The listing builds one solid part. Answer for the finished solid, in the listing's coordinates (mm). A direction names the side the tool comes from. Give positions to 0.01 mm unless a question says otherwise; leave off trailing zeros. Loops run counter-clockwise (first coordinate to the right, second up) from the corner with the lowest first, then second, coordinate; pieces in that order, holes last. Notation, with made-up numbers: M 85.5,-33 L 128.5,-33 A5 cw 128.5,-27 Z; hole C 26,71 d4. An arc over 180 degrees is marked long. Return JSON: item names as keys, results as strings.
Autodesk Inventor part; units mm, degrees
ref_plane "작업 평면1" through (0, 0, 0) normal (0, 0, 1) x (1, 0, 0)
ref_plane "YZ Plane" through (0, 0, 0) normal (1, 0, 0) x (0, 1, 0)
ref_plane "XZ Plane" through (0, 0, 0) normal (0, 1, 0) x (-1, 0, 0)
sketch "스케치1" plane through (0, 0, 0) normal (0, 0, 1) x (1, 0, 0)
  line L0 (0, 0) -> (24, 0)
  line L1 (24, 0) -> (24, -24)
  line L2 (24, -24) -> (0, -24)
  line L3 (0, -24) -> (0, 0)
  circle A0 centre (12, -12) radius 2.5
  dimension "d0" = 24
  dimension "d1" = 24
  dimension "d2" = 5
  dimension "d3" = 12
  dimension "d4" = 12
extrude "돌출1" add sketch "스케치1" along normal mid plane 35
fillet "모깎기1" radius 20 1 edges at (0, -24, 0)
chamfer "모따기1" distance 2 angle 45 4 edges at (12, 0, 17.5) (12, 0, -17.5) (24, -12, 17.5) (24, -12, -17.5)
ref_plane "작업 평면1" through (0, 0, 0) normal (0, 0, 1) x (1, 0, 0)
sketch "스케치2" plane through (0, 0, 0) normal (0, 0, 1) x (1, 0, 0)
  line L0 (24, -24) -> (24, 0)
  line L1 (24, 0) -> (20, 0)
  line L2 (20, 0) -> (20, -4)
  line L3 (20, -4) -> (24, -4)
  line L4 (24, -4) -> (24, 0)
  line L5 (0, 0) -> (0, -2)
  line L6 (0, 0) -> (4, 0)
  line L7 (4, 0) -> (4, -4)
  line L8 (4, -4) -> (0, -4)
  line L9 (0, -4) -> (0, 0)
  line L10 (22, -24) -> (24, -24)
  line L11 (24, -24) -> (20, -24)
  line L12 (20, -24) -> (20, -20)
  line L13 (20, -20) -> (24, -20)
  line L14 (24, -20) -> (24, -24)
  line L15 (22, -2) -> (24, 0)
  line L16 (24, 0) -> (0, 0)
  line L17 (0, 0) -> (0, -24)
  line L18 (0, -24) -> (24, -24)
  line L19 (24, -24) -> (24, 0)
  dimension "d11" = 4
  dimension "d12" = 4
  dimension "d13" = 4
  dimension "d14" = 4
  dimension "d15" = 4
extrude "돌출2" cut sketch "스케치2" along normal mid plane 27 contours L13 L12 L18 L17 L8 L7 L16 L2 L3 L0
properties part number "16-1"
(1) The part is cut by section C-C (y = -19). Determine the outline of the cut face in (x, z).
Values follow:
{"outline": "M 6.77,-17.5 L 22,-17.5 L 24,-15.5 L 24,-13.5 L 6.77,-13.5 Z; M 6.77,13.5 L 24,13.5 L 24,15.5 L 22,17.5 L 6.77,17.5 Z"}
(2) Given pin 1 (6 mm diameter, centred on x = 6, z = -8.5, fed in from -Y); pin 2 (4 mm diameter, centred on x = 12, y = -12, fed in from +Z); pin 3 (3 mm diameter, centred on y = -21.5, z = 0, fed in from -X), each flat-ended and moving along its own axis, determine where each tip first touches the part or whether it passes through.
Values follow:
{"pin 1": "y = -4", "pin 2": "through", "pin 3": "x = 20"}
(3) Determine the mould class of faces 4 (the flat face through (14, -9, -13.5)), 5 (the cylindrical face through (5.703, -17.986, 15.528)), 6 (the flat face through (23, -11.8, 16.5)) for opening direction Z: released by +Z, released by -Z, zero draft, split by the parting line, or undercut.
Values follow:
{"face 4": "undercut", "face 5": "zero draft", "face 6": "released by +Z"}
(4) Straight lines are drawn through the part: line 1 along Z through (x, y) = (7.75, -19.5); line 2 along Y through (x, z) = (2.25, 12.5); line 3 along Y through (x, z) = (12, -16.4). For each, find the intervals that lie inside material, in ascending order.
Values follow:
{"line 1": "-17.5 to -13.5, 13.5 to 17.5", "line 2": "-4 to 0", "line 3": "-22.33 to -14.5, -9.5 to -0.9"}
(5) The part is cut by section D-D (x = 4.5). Determine the outline of the cut face in (y, z).
Values follow:
{"outline": "M -16.64,-17.5 L -2,-17.5 L 0,-15.5 L 0,-13.5 L -16.64,-13.5 Z; M -16.64,13.5 L 0,13.5 L 0,15.5 L -2,17.5 L -16.64,17.5 Z"}
(6) The part is cut by section A-A (z = -6). Determine the outline of the cut face in (x, y), and give its area (3 significant figures).
Values follow:
{"outline": "M 0,-4 L 4,-4 L 4,0 L 0,0 Z; M 20,-24 L 24,-24 L 24,-20 L 20,-20 Z; M 20,-4 L 24,-4 L 24,0 L 20,0 Z", "area": "48.0 mm²"}
(7) A tool of negligible diameter and unlimited length cuts with its end or side. For faces 1 (the flat face through (4, -2, 0)), 2 (the flat face through (2, -4, 0)), 3 (the flat face through (22, -20, 0)), from which of +Z, -Z, +X, -X, +Y, -Y can it reach the whole face along a straight path? Write none if from no direction.
Values follow:
{"face 1": "+Y, -Y", "face 2": "+X, -X, -Y", "face 3": "+X, -X"}
(8) The part is cut by section B-B (x = 12). Determine the outline of the cut face in (y, z).
Values follow:
{"outline": "M -22.33,-17.5 L -14.5,-17.5 L -14.5,-13.5 L -22.33,-13.5 Z; M -22.33,13.5 L -14.5,13.5 L -14.5,17.5 L -22.33,17.5 Z; M -9.5,-17.5 L -2,-17.5 L 0,-15.5 L 0,-13.5 L -9.5,-13.5 Z; M -9.5,13.5 L 0,13.5 L 0,15.5 L -2,17.5 L -9.5,17.5 Z"}
